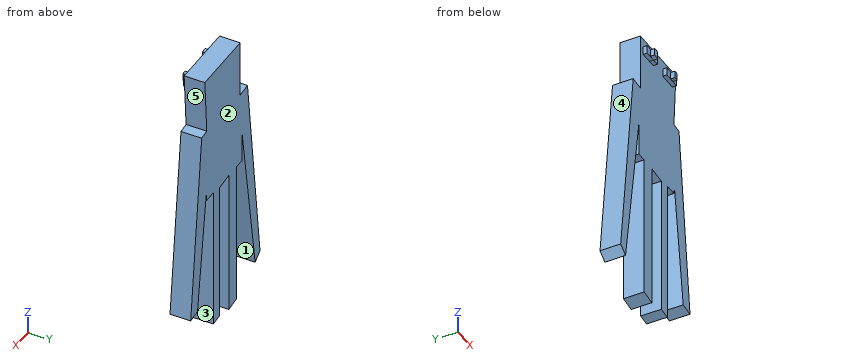
```python
from build123d import *

# Parameters (mm, degrees)
F1_DEPTH = 5
F3_DEPTH = 6
F4_W     = 1.006404
F4_H     = 1.725264
F5_DEPTH = 7


with BuildPart() as f1:
    # F0 (on Front) → F1 (new body)
    with BuildSketch(Plane.XZ):
        Polygon((-9.354408, 7.877359), (-12.614951, 8.239642), (-18.230332, -39.76281), (-16.056636, -41.393083), (-10.078973, -2.266556), (-10.078973, -10.236774), (-7.724135, -10.236774), (-4.225735, -10.236774), (2.712137, -10.236774), (5.680322, -10.236774), (5.927842, -8.616642), (9.846571, -37.22683), (12.894985, -37.692559), (7.959375, 7.895558), (5.680322, 8.243747), (6.543175, 21.825243), (-9.354408, 21.825243), align=None)
        Polygon((-4.225735, -10.236774), (-7.724135, -10.236774), (-7.724135, -45.559332), (-4.225735, -46.09381), align=None)
        Polygon((2.712137, -10.236774), (-4.225735, -10.236774), (0, -10.731105), (0, -45.015905), (2.712137, -45.333174), align=None)
    extrude(amount=F1_DEPTH)

    # F2 (on Front) → F3 (join)
    with BuildSketch(Plane.XZ):
        Polygon((-3.647329, 19.689403), (-8.165929, 19.729748), (-8.165929, 17.712517), (-3.647329, 17.712517), align=None)
        Polygon((4.986425, 17.752862), (4.986425, 19.366648), (4.986425, 19.691204), (0.669532, 19.729748), (0.669532, 17.791406), align=None)
    extrude(amount=F3_DEPTH)

    # F4 (on Front) → F5 (join)
    with BuildSketch(Plane.XZ):
        Polygon((-6.671616, 19.56287), (-6.671616, 17.837606), (-5.305782, 17.693834), (-5.305782, 19.56287), align=None)
        with Locations((2.889219, 18.700238)):
            Rectangle(F4_W, F4_H)
    extrude(amount=F5_DEPTH)


solid = f1.part
```
Can you work these out from the model? Positions are in its coordinate system, mm. Face numbers are marked on the shaded views. A direction names the side the tool comes from. Round coordinates to 2 decimals unless told otherwise and drop trailing zeros. Loops run counter-clockwise (first coordinate to the right, second up) from the corner with the lowest first, then second, coordinate; pieces in that order, holes last. Notation, with made-up numbers: M 38,-38 L 70,-38 A23 ccw 70,-20 Z; hole C -16,26.5 d10. An arc over 180 degrees is marked long. Answer as a JSON object with one key per item and string values. Group by question number.
Q1. Imagine slicing it at B-B, the plane y = -2.5. Please give me the cut outline in (x, z).
Q2. Imagine slicing it at C-C, the plane z = -32.5. Please give me the cut outline in (x, y).
Q3. On a 3-axis mill with a long thin cutter (end or side, diameter ignored), from which of +Z, -Z, +X, -X, +Y, -Y can I reach the whole of each face in a straight line? I mean the marked faces 3, 4 and 5. Say none if no direction works.
Q4. Imagine slicing it at D-D, the plane x = -15. Please give me the cut outline in (y, z), then the cut area to 3 significant figures.
Q5. Imagine slicing it at A-A, the plane z = -42. Please give me the cut outline in (x, y).
Q6. We'd pull the mould along Y, two halves only. Please class the marked faces 1 and 2: +Y half, -Y half, draft (parallel to the pull), parting line (faces both ways), or undercut.
Q7. Please list where these lines run through material, in increasing order: L1, parallel to X at y = -4.5, z = -23.5; L2, parallel to X at y = -1.75, z = -23; L3, parallel to Y at x = 3, z = 2.
Q8. Will these pins go through, and if not, where does the flat tip stop? pin 1 (1.5 mm diameter, centred on x = 7, y = -6, fed in from +Z); pin 2 (2.5 mm diameter, centred on y = -2.5, z = -31.5, fed in from -X); pin 3 (6 mm diameter, centred on x = -4.5, z = -38, fed in from -Y); pin 4 (3.5 mm diameter, centred on x = 3.5, y = -3, fed in from -Z).
Findings:
{
 "1": {"outline": "M -18.23,-39.76 L -16.06,-41.39 L -10.08,-2.27 L -10.08,-10.24 L -7.72,-10.24 L -7.72,-45.56 L -4.23,-46.09 L -4.23,-10.24 L 0,-10.73 L 0,-45.02 L 2.71,-45.33 L 2.71,-10.24 L 5.68,-10.24 L 5.93,-8.62 L 9.85,-37.23 L 12.89,-37.69 L 7.96,7.9 L 5.68,8.24 L 6.54,21.83 L -9.35,21.83 L -9.35,7.88 L -12.61,8.24 Z"},
 "2": {"outline": "M -17.38,-5 L -14.7,-5 L -14.7,0 L -17.38,0 Z; M -7.72,-5 L -4.23,-5 L -4.23,0 L -7.72,0 Z; M 0,-5 L 2.71,-5 L 2.71,0 L 0,0 Z; M 9.2,-5 L 12.33,-5 L 12.33,0 L 9.2,0 Z"},
 "3": {"face 3": "-Z, +Y, -Y", "face 4": "+Z, -X, +Y, -Y", "face 5": "+X, +Y, -Y"},
 "4": {"outline": "M -5,-34.48 L 0,-34.48 L 0,-12.15 L -5,-12.15 Z", "area": "112 mm2"},
 "5": {"outline": "M -7.72,-5 L -4.23,-5 L -4.23,0 L -7.72,0 Z; M 0,-5 L 2.71,-5 L 2.71,0 L 0,0 Z"},
 "6": {"face 1": "draft", "face 2": "+Y half"},
 "7": {"L1": "x = -16.33 to -13.32, -7.72 to -4.23, 0 to 2.71, 7.97 to 11.36", "L2": "x = -16.27 to -13.25, -7.72 to -4.23, 0 to 2.71, 7.9 to 11.3", "L3": "y = -5 to 0"},
 "8": {"pin 1": "passes through", "pin 2": "stops at x = -17.41", "pin 3": "stops at y = -5", "pin 4": "stops at z = -45.33"}
}
